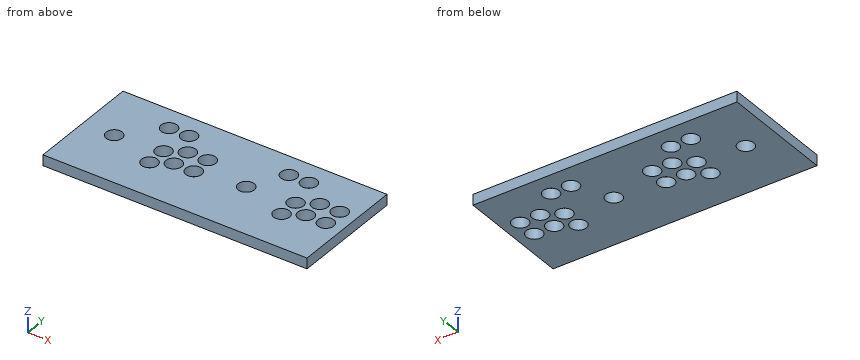
from build123d import *

# Parameters (mm, degrees)
F0_W     = 469.9
F0_H     = 203.2
F0_W_2   = 79.375
F0_H_2   = 88.9
F0_R     = 14.2875
F1_DEPTH = 19.05


with BuildPart() as f1:
    # F0 (on Top) → F1 (new body)
    with BuildSketch(Plane.XY):
        Rectangle(F0_W, F0_H)
        with Locations((-179.3875, 0)):
            Rectangle(F0_W_2, F0_H_2, mode=Mode.SUBTRACT)
        with Locations((-96.518363, -28.575)):
            Circle(F0_R, mode=Mode.SUBTRACT)
        with Locations((-65.7225, -10.795)):
            Circle(F0_R, mode=Mode.SUBTRACT)
        with Locations((-30.1625, -10.795)):
            Circle(F0_R, mode=Mode.SUBTRACT)
        with Locations((55.5625, 0)):
            Rectangle(F0_W_2, F0_H_2, mode=Mode.SUBTRACT)
        with Locations((138.431637, -28.575)):
            Circle(F0_R, mode=Mode.SUBTRACT)
        with Locations((169.2275, -10.795)):
            Circle(F0_R, mode=Mode.SUBTRACT)
        with Locations((204.7875, -10.795)):
            Circle(F0_R, mode=Mode.SUBTRACT)
        with Locations((-96.518363, 6.985)):
            Circle(F0_R, mode=Mode.SUBTRACT)
        with Locations((-65.7225, 24.765)):
            Circle(F0_R, mode=Mode.SUBTRACT)
        with Locations((-30.1625, 24.765)):
            Circle(F0_R, mode=Mode.SUBTRACT)
        with Locations((-124.46, 60.96)):
            Circle(F0_R, mode=Mode.SUBTRACT)
        with Locations((-88.9, 60.96)):
            Circle(F0_R, mode=Mode.SUBTRACT)
        with Locations((138.431637, 6.985)):
            Circle(F0_R, mode=Mode.SUBTRACT)
        with Locations((169.2275, 24.765)):
            Circle(F0_R, mode=Mode.SUBTRACT)
        with Locations((204.7875, 24.765)):
            Circle(F0_R, mode=Mode.SUBTRACT)
        with Locations((88.9, 60.96)):
            Circle(F0_R, mode=Mode.SUBTRACT)
        with Locations((124.46, 60.96)):
            Circle(F0_R, mode=Mode.SUBTRACT)
        with Locations((-179.3875, 0)):
            Rectangle(F0_W_2, F0_H_2)
        with Locations((-179.3875, 0)):
            Circle(F0_R, mode=Mode.SUBTRACT)
        with Locations((55.5625, 0)):
            Rectangle(F0_W_2, F0_H_2)
        with Locations((55.5625, 0)):
            Circle(F0_R, mode=Mode.SUBTRACT)
    extrude(amount=F1_DEPTH)


solid = f1.part
Part model, mm, in its own coordinate system. Coordinates: 2 decimals unless noted, no trailing zeros. Order: outer loops, then holes, each group sorted by start corner. A loop starts at its lowest first (then second) coordinate and runs counter-clockwise, first axis right, second up. Notation, with made-up numbers: M -25.75,70.25 L 18.25,70.25 A25 ccw 18.25,82.25 Z; hole C -17,55 d3. An arc over 180 degrees is marked long. Use a Markdown table: item, result.
(1) Cut at A-A on x = -124.46. Write the cut outline in (y, z), then the cut area to 3 significant figures.
A:
| item | result |
|---|---|
| outline | M -101.6,0 L 46.67,0 L 46.67,19.05 L -101.6,19.05 Z; M 75.25,0 L 101.6,0 L 101.6,19.05 L 75.25,19.05 Z |
| area | 3,330 mm^2 |
(2) Flat gauge pin, fed straight in: pin 1 (17 mm diameter, centred on x = 204.79, y = 24.76, fed in from -Z). Where does the tip first touch, or does it go through?
A:
| item | result |
|---|---|
| pin 1 | passes through |
(3) Cut at C-C on x = -189.5. Write the cut outline in (y, z).
A:
| item | result |
|---|---|
| outline | M -101.6,0 L -10.09,0 L -10.09,19.05 L -101.6,19.05 Z; M 10.09,0 L 101.6,0 L 101.6,19.05 L 10.09,19.05 Z |
(4) Probe L1, parallel to X at y = 28.5, z = 14; L2, parallel to X at y = 22, z = 9.5; L3, parallel to Y at x = 132, z = 10.5. List the from-to ranges inside material, lowest first.
A:
| item | result |
|---|---|
| L1 | x = -234.95 to -79.51, -51.93 to -43.95, -16.37 to 155.44, 183.02 to 191, 218.58 to 234.95 |
| L2 | x = -234.95 to -79.74, -51.71 to -44.18, -16.15 to 155.21, 183.24 to 190.77, 218.8 to 234.95 |
| L3 | y = -101.6 to -41.33, -15.82 to -5.77, 19.74 to 48.82, 73.1 to 101.6 |
(5) Cut at B-B on z = 3. State how many separate pieces and enclosed holes the cut face has, then the cut area to 3 significant figures.
A:
| item | result |
|---|---|
| separate pieces | 1 |
| enclosed holes | 18 |
| area | 83,900 mm^2 |
